Input: part model. Units: mm. Frame: model coordinates. A direction names the side the tool comes from. Round coordinates to 2 decimals unless told otherwise and drop trailing zeros. Loops run counter-clockwise (first coordinate to the right, second up) from the corner with the lowest first, then second, coordinate; pieces in that order, holes last.
(1) Cut plane A-A, the plane z = 21. Output: boundary loops of the cut face in (x, y), and give its area (3 significant figures).
(2) Cut plane D-D, the plane y = 48.5. Output: boundary loops of the cut face in (x, z), and give its area (3 significant figures).
(3) Access query for faces 1 (the face through (28, 55, 33)), 2 (the face through (26, 1, 36)), 3 (the face through (26.521, 55.797, 37.859)), 4 (the face through (25, 55, 33)), 5 (the face through (0, 11, 35)). Directions: +Z, -Z, +X, -X, +Y, -Y. A direction counts if a zero-diameter tool reaches every point of the face in a straight line with its end or side. Return the directions, or none.
(4) Draft query along Y for faces 6 (the face through (26, 25, 2)), 7 (the face through (26, 51, 31)), 8 (the face through (26, 0, 35)). Return one class per face: released by +Y, released by -Y, zero draft, split by the parting line, or undercut.
(5) First-contact query: pin 1 Ø2 at (x, y) = (46.5, 44.5) entering from -Z; pin 2 Ø6 at (y, z) = (42.5, 62.5) entering from -X; pin 3 Ø6 at (y, z) = (12, 62.5) entering from -X; pin 4 Ø10 at (x, y) = (17.5, 35.5) entering from +Z. Flat tips, straight axial feed; report the tip coordinate or a pass-through.
(6) Cut plane C-C, the plane x = 43. Output: boundary loops of the cut face in (y, z), and give its area (3 significant figures).
(7) Cut plane B-B, the plane y = 10. Output: boundary loops of the cut face in (x, z), and give its area (3 significant figures).
(8) Line query: line 1 (Y direction, x = 26, z = 35); line 2 (Y direction, x = 27, z = 21); line 3 (X direction, y = 24.5, z = 19). Output: solid intervals per line, ascending.
from build123d import *

# Parameters (mm, degrees)
ESQUISSE1_W             = 53
ESQUISSE1_H             = 50
BOSS_EXTRU_1_DEPTH      = 70
ESQUISSE5_W             = 3
ESQUISSE5_H             = 8
BOSS_EXTRU_2_DEPTH      = 7
CONG_1_R                = 4
CONG_2_R                = 27
ESQUISSE8_R             = 2.5
ENL_V_MAT_EXTRU_3_DEPTH = 7
ENL_V_MAT_EXTRU_4_DEPTH = 68


# Some blends are built 0.0001 mm under size
with BuildPart() as part:
    # Esquisse1 → Boss.-Extru.1 (new body)
    with BuildSketch(Plane.XY):
        with Locations((26.5, 25)):
            Rectangle(ESQUISSE1_W, ESQUISSE1_H)
    extrude(amount=BOSS_EXTRU_1_DEPTH)

    # Esquisse5 → Boss.-Extru.2 (add)
    with BuildSketch(Plane(origin=(0, 50, 0), x_dir=(1, 0, 0), z_dir=(0, 1, 0))):
        with Locations((26.5, -35)):
            Rectangle(ESQUISSE5_W, ESQUISSE5_H)
    extrude(amount=BOSS_EXTRU_2_DEPTH)

    # Congé1
    cong_1_edges = [part.edges().sort_by_distance(p)[0] for p in [
        (26.5, 57, 31),
        (26.5, 57, 39),
    ]]
    fillet(cong_1_edges, radius=CONG_1_R - 0.0001)  # a hair under: the kernel refuses the full size

    # Congé2
    # the kernel refuses this fillet: 27 mm, written as the material it takes off along each edge
    with BuildSketch(Plane(origin=(0, 50, -67.5), x_dir=(1, 0, 0), z_dir=(0, 0, 1))) as cong_2_piece_1_section:
        with BuildLine():
            CenterArc((CONG_2_R, -CONG_2_R), CONG_2_R, 90, 90)
            Line((0, -CONG_2_R), (0, 0))
            Line((0, 0), (CONG_2_R, 0))
        make_face()
    cong_2_piece_1 = extrude(amount=205, mode=Mode.PRIVATE)
    cong_2_piece_1 = split(cong_2_piece_1, bisect_by=Plane(origin=(25, 50.257211281, -18.25), z_dir=(1, 0, 0)), keep=Keep.TOP, mode=Mode.PRIVATE)
    cong_2_piece_1 = split(cong_2_piece_1, bisect_by=Plane(origin=(25.978114042, 50.257211281, 31), z_dir=(0, 0, -1)), keep=Keep.TOP, mode=Mode.PRIVATE)
    add(cong_2_piece_1, mode=Mode.SUBTRACT)
    with BuildSketch(Plane(origin=(0, 50, -67.5), x_dir=(1, 0, 0), z_dir=(0, 0, 1))) as cong_2_piece_2_section:
        with BuildLine():
            CenterArc((CONG_2_R, -CONG_2_R), CONG_2_R, 90, 90)
            Line((0, -CONG_2_R), (0, 0))
            Line((0, 0), (CONG_2_R, 0))
        make_face()
    cong_2_piece_2 = extrude(amount=205, mode=Mode.PRIVATE)
    cong_2_piece_2 = split(cong_2_piece_2, bisect_by=Plane(origin=(25, 43.848394797, -18.25), z_dir=(-1, 0, 0)), keep=Keep.TOP, mode=Mode.PRIVATE)
    cong_2_piece_2 = split(cong_2_piece_2, bisect_by=Plane(origin=(5.991236712, 43.848394797, 31), z_dir=(0, 0, -1)), keep=Keep.TOP, mode=Mode.PRIVATE)
    add(cong_2_piece_2, mode=Mode.SUBTRACT)
    with BuildSketch(Plane(origin=(0, 50, -67.5), x_dir=(1, 0, 0), z_dir=(0, 0, 1))) as cong_2_piece_3_section:
        with BuildLine():
            CenterArc((CONG_2_R, -CONG_2_R), CONG_2_R, 90, 90)
            Line((0, -CONG_2_R), (0, 0))
            Line((0, 0), (CONG_2_R, 0))
        make_face()
    cong_2_piece_3 = extrude(amount=205, mode=Mode.PRIVATE)
    cong_2_piece_3 = split(cong_2_piece_3, bisect_by=Plane(origin=(25, 43.848394797, 35), z_dir=(-1, 0, 0)), keep=Keep.TOP, mode=Mode.PRIVATE)
    cong_2_piece_3 = split(cong_2_piece_3, bisect_by=Plane(origin=(5.991236712, 43.848394797, 31), z_dir=(0, 0, 1)), keep=Keep.TOP, mode=Mode.PRIVATE)
    cong_2_piece_3 = split(cong_2_piece_3, bisect_by=Plane(origin=(5.991236712, 43.848394797, 39), z_dir=(0, 0, -1)), keep=Keep.TOP, mode=Mode.PRIVATE)
    add(cong_2_piece_3, mode=Mode.SUBTRACT)
    with BuildSketch(Plane(origin=(0, 50, -67.5), x_dir=(1, 0, 0), z_dir=(0, 0, 1))) as cong_2_piece_4_section:
        with BuildLine():
            CenterArc((CONG_2_R, -CONG_2_R), CONG_2_R, 90, 90)
            Line((0, -CONG_2_R), (0, 0))
            Line((0, 0), (CONG_2_R, 0))
        make_face()
    cong_2_piece_4 = extrude(amount=205, mode=Mode.PRIVATE)
    cong_2_piece_4 = split(cong_2_piece_4, bisect_by=Plane(origin=(25, 50.257211281, 88.25), z_dir=(1, 0, 0)), keep=Keep.TOP, mode=Mode.PRIVATE)
    cong_2_piece_4 = split(cong_2_piece_4, bisect_by=Plane(origin=(25.978114042, 50.257211281, 39), z_dir=(0, 0, 1)), keep=Keep.TOP, mode=Mode.PRIVATE)
    add(cong_2_piece_4, mode=Mode.SUBTRACT)
    with BuildSketch(Plane(origin=(0, 50, -67.5), x_dir=(1, 0, 0), z_dir=(0, 0, 1))) as cong_2_piece_5_section:
        with BuildLine():
            CenterArc((CONG_2_R, -CONG_2_R), CONG_2_R, 90, 90)
            Line((0, -CONG_2_R), (0, 0))
            Line((0, 0), (CONG_2_R, 0))
        make_face()
    cong_2_piece_5 = extrude(amount=205, mode=Mode.PRIVATE)
    cong_2_piece_5 = split(cong_2_piece_5, bisect_by=Plane(origin=(25, 43.848394797, 88.25), z_dir=(-1, 0, 0)), keep=Keep.TOP, mode=Mode.PRIVATE)
    cong_2_piece_5 = split(cong_2_piece_5, bisect_by=Plane(origin=(5.991236712, 43.848394797, 39), z_dir=(0, 0, 1)), keep=Keep.TOP, mode=Mode.PRIVATE)
    add(cong_2_piece_5, mode=Mode.SUBTRACT)
    with BuildSketch(Plane(origin=(53, 50, -67.5), x_dir=(-1, 0, 0), z_dir=(0, 0, 1))) as cong_2_piece_6_section:
        with BuildLine():
            CenterArc((CONG_2_R, CONG_2_R), CONG_2_R, 180, 90)
            Line((0, CONG_2_R), (0, 0))
            Line((0, 0), (CONG_2_R, 0))
        make_face()
    cong_2_piece_6 = extrude(amount=205, mode=Mode.PRIVATE)
    cong_2_piece_6 = split(cong_2_piece_6, bisect_by=Plane(origin=(27.021885958, 50.257211281, 31), z_dir=(0, 0, -1)), keep=Keep.TOP, mode=Mode.PRIVATE)
    cong_2_piece_6 = split(cong_2_piece_6, bisect_by=Plane(origin=(28, 50.257211281, -18.25), z_dir=(-1, 0, 0)), keep=Keep.TOP, mode=Mode.PRIVATE)
    add(cong_2_piece_6, mode=Mode.SUBTRACT)
    with BuildSketch(Plane(origin=(53, 50, -67.5), x_dir=(-1, 0, 0), z_dir=(0, 0, 1))) as cong_2_piece_7_section:
        with BuildLine():
            CenterArc((CONG_2_R, CONG_2_R), CONG_2_R, 180, 90)
            Line((0, CONG_2_R), (0, 0))
            Line((0, 0), (CONG_2_R, 0))
        make_face()
    cong_2_piece_7 = extrude(amount=205, mode=Mode.PRIVATE)
    cong_2_piece_7 = split(cong_2_piece_7, bisect_by=Plane(origin=(47.008763288, 43.848394797, 31), z_dir=(0, 0, -1)), keep=Keep.TOP, mode=Mode.PRIVATE)
    cong_2_piece_7 = split(cong_2_piece_7, bisect_by=Plane(origin=(28, 43.848394797, -18.25), z_dir=(1, 0, 0)), keep=Keep.TOP, mode=Mode.PRIVATE)
    add(cong_2_piece_7, mode=Mode.SUBTRACT)
    with BuildSketch(Plane(origin=(53, 50, -67.5), x_dir=(-1, 0, 0), z_dir=(0, 0, 1))) as cong_2_piece_8_section:
        with BuildLine():
            CenterArc((CONG_2_R, CONG_2_R), CONG_2_R, 180, 90)
            Line((0, CONG_2_R), (0, 0))
            Line((0, 0), (CONG_2_R, 0))
        make_face()
    cong_2_piece_8 = extrude(amount=205, mode=Mode.PRIVATE)
    cong_2_piece_8 = split(cong_2_piece_8, bisect_by=Plane(origin=(47.008763288, 43.848394797, 31), z_dir=(0, 0, 1)), keep=Keep.TOP, mode=Mode.PRIVATE)
    cong_2_piece_8 = split(cong_2_piece_8, bisect_by=Plane(origin=(28, 43.848394797, 35), z_dir=(1, 0, 0)), keep=Keep.TOP, mode=Mode.PRIVATE)
    cong_2_piece_8 = split(cong_2_piece_8, bisect_by=Plane(origin=(47.008763288, 43.848394797, 39), z_dir=(0, 0, -1)), keep=Keep.TOP, mode=Mode.PRIVATE)
    add(cong_2_piece_8, mode=Mode.SUBTRACT)
    with BuildSketch(Plane(origin=(53, 50, -67.5), x_dir=(-1, 0, 0), z_dir=(0, 0, 1))) as cong_2_piece_9_section:
        with BuildLine():
            CenterArc((CONG_2_R, CONG_2_R), CONG_2_R, 180, 90)
            Line((0, CONG_2_R), (0, 0))
            Line((0, 0), (CONG_2_R, 0))
        make_face()
    cong_2_piece_9 = extrude(amount=205, mode=Mode.PRIVATE)
    cong_2_piece_9 = split(cong_2_piece_9, bisect_by=Plane(origin=(28, 50.257211281, 88.25), z_dir=(-1, 0, 0)), keep=Keep.TOP, mode=Mode.PRIVATE)
    cong_2_piece_9 = split(cong_2_piece_9, bisect_by=Plane(origin=(27.021885958, 50.257211281, 39), z_dir=(0, 0, 1)), keep=Keep.TOP, mode=Mode.PRIVATE)
    add(cong_2_piece_9, mode=Mode.SUBTRACT)
    with BuildSketch(Plane(origin=(53, 50, -67.5), x_dir=(-1, 0, 0), z_dir=(0, 0, 1))) as cong_2_piece_10_section:
        with BuildLine():
            CenterArc((CONG_2_R, CONG_2_R), CONG_2_R, 180, 90)
            Line((0, CONG_2_R), (0, 0))
            Line((0, 0), (CONG_2_R, 0))
        make_face()
    cong_2_piece_10 = extrude(amount=205, mode=Mode.PRIVATE)
    cong_2_piece_10 = split(cong_2_piece_10, bisect_by=Plane(origin=(28, 43.848394797, 88.25), z_dir=(1, 0, 0)), keep=Keep.TOP, mode=Mode.PRIVATE)
    cong_2_piece_10 = split(cong_2_piece_10, bisect_by=Plane(origin=(47.008763288, 43.848394797, 39), z_dir=(0, 0, 1)), keep=Keep.TOP, mode=Mode.PRIVATE)
    add(cong_2_piece_10, mode=Mode.SUBTRACT)

    # Esquisse8 → Enlèv. mat.-Extru.3 (cut)
    with BuildSketch(Plane.ZY.offset(-25)):
        with Locations((35, 53)):
            Circle(ESQUISSE8_R)
    extrude(amount=-ENL_V_MAT_EXTRU_3_DEPTH, mode=Mode.SUBTRACT)

    # Esquisse9 → Enlèv. mat.-Extru.4 (cut)
    with BuildSketch(Plane.XY.offset(70)):
        with BuildLine():
            Line((2, 1), (51, 1))
            Line((51, 1), (51, 23))
            ThreePointArc((51, 23), (43.829843545, 40.318386839), (26.516202227, 47.499994643))
            ThreePointArc((26.516202227, 47.499994643), (9.181613161, 40.329843545), (2, 23))
            Line((2, 23), (2, 1))
        make_face()
    extrude(amount=-ENL_V_MAT_EXTRU_4_DEPTH, mode=Mode.SUBTRACT)


solid = part.part
Reported:
1. outline: (0, 0) - (53, 0) - (53, 23) arc R27 ccw to (26.5, 50) arc R27 ccw to (0, 23) - close; hole (2, 1) - (51, 1) - (51, 23) arc R24.5 ccw to (2, 23) - close
1. area: 316 mm2
2. outline: (18.13, 0) - (34.87, 0) - (34.87, 70) - (18.13, 70) - close
2. area: 1,170 mm2
3. face 1: +Z, -Z, +X, +Y
3. face 2: +Z
3. face 3: +Z, +X, -X, +Y
3. face 4: +Z, -Z, -X, +Y
3. face 5: +Z, -Z, -X, +Y, -Y
4. face 6: undercut
4. face 7: zero draft
4. face 8: released by -Y
5. pin 1: passes through
5. pin 2: stops at x = 5.63
5. pin 3: stops at x = 0
5. pin 4: stops at z = 2
6. outline: (0, 0) - (43.98, 0) - (43.98, 70) - (41.11, 70) - (41.11, 2) - (1, 2) - (1, 70) - (0, 70) - close
6. area: 351 mm2
7. outline: (0, 0) - (53, 0) - (53, 70) - (51, 70) - (51, 2) - (2, 2) - (2, 70) - (0, 70) - close
7. area: 378 mm2
8. line 1: y = 0 to 1, 47.49 to 50.5, 55.5 to 57
8. line 2: y = 0 to 1, 47.49 to 49.98
8. line 3: x = 0.04 to 2.05, 50.95 to 52.96
